Study the drawing (mm; zero at the part's minimum x, y, z) and answer. A direction names the side the tool comes from. Round coordinates to 2 decimals unless told otherwise and drop trailing zeros. Write each loop counter-clockwise with the first axis right and the second up, starting at its lowest first coordinate (ties: lowest second). Pieces come first, ordered by that corner, then holes. Notation, with made-up numbers: (-34.5, 71.25) - (-2.5, 71.25) arc R20 ccw to (-2.5, 107.25) - close; hole circle Ø1 at (75, 6). An arc over 180 degrees is marked (long way). Use one line per item in the form item = value. Start each with the question number.
1) The part is cut by section C-C, the plane x = 1.1. Give the vertices of the cut face in (y, z).
2) The part is cut by section D-D, the plane y = 0.7. Give the vertices of the cut face in (x, z), plus the area to 3 significant figures.
3) For the marked faces 5, 6 and 7, determine the directions among +Z, -Z, +X, -X, +Y, -Y from which every point of the face is accessible in a straight line to the end or side of a thin tool.
4) The part is cut by section B-B, the plane y = 1.25. Give the vertices of the cut face in (x, z) (3 decimals), plus the area to 3 significant figures.
5) The part is cut by section A-A, the plane z = 1. Give the vertices of the cut face in (x, y) (3 decimals), plus the area to 3 significant figures.
6) Consider line 1 along Z through (x, y) = (2.7, 1.2); line 2 along Z through (x, y) = (3.45, 1.9); line 3 along X through (y, z) = (1.15, 2.5). Determine where each line is inside the solid, lowest interval first. Write a range as from..to.
7) For a pull along X with two mould halves and no side action, classify the marked faces 1, 2, 3 and 4 as released by +X, released by -X, zero draft, split by the parting line, or undercut.
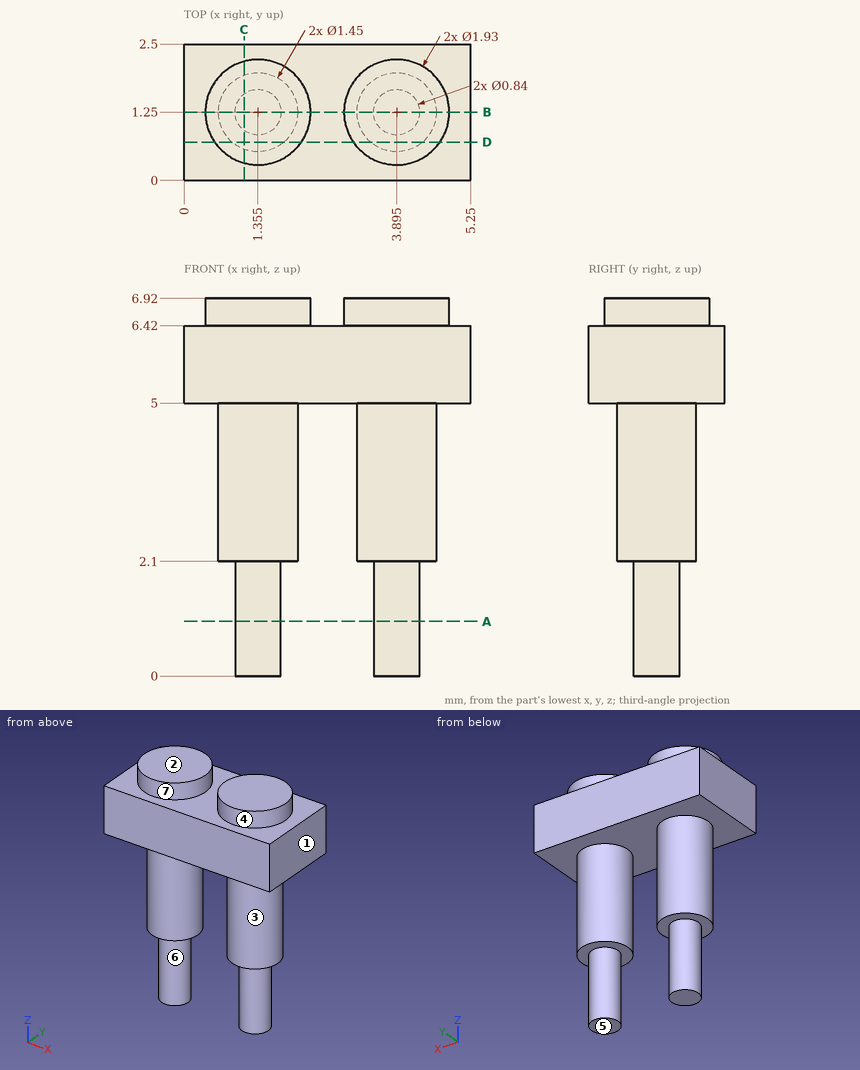
Geometry results:
q1.outline = (0, 5) - (0.57, 5) - (0.57, 2.1) - (0.92, 2.1) - (0.92, 0) - (1.58, 0) - (1.58, 2.1) - (1.93, 2.1) - (1.93, 5) - (2.5, 5) - (2.5, 6.42) - (2.18, 6.42) - (2.18, 6.92) - (0.32, 6.92) - (0.32, 6.42) - (0, 6.42) - close
q2.outline = (0, 5) - (0.88, 5) - (0.88, 2.1) - (1.83, 2.1) - (1.83, 5) - (3.42, 5) - (3.42, 2.1) - (4.37, 2.1) - (4.37, 5) - (5.25, 5) - (5.25, 6.42) - (4.69, 6.42) - (4.69, 6.92) - (3.1, 6.92) - (3.1, 6.42) - (2.15, 6.42) - (2.15, 6.92) - (0.56, 6.92) - (0.56, 6.42) - (0, 6.42) - close
q2.area = 14.5 mm2
q3.face_5 = -Z, +X, -X, +Y, -Y
q3.face_6 = -Z
q3.face_7 = +Z
q4.outline = (0, 5) - (0.63, 5) - (0.63, 2.1) - (0.935, 2.1) - (0.935, 0) - (1.775, 0) - (1.775, 2.1) - (2.08, 2.1) - (2.08, 5) - (3.17, 5) - (3.17, 2.1) - (3.475, 2.1) - (3.475, 0) - (4.315, 0) - (4.315, 2.1) - (4.62, 2.1) - (4.62, 5) - (5.25, 5) - (5.25, 6.42) - (4.86, 6.42) - (4.86, 6.92) - (2.93, 6.92) - (2.93, 6.42) - (2.32, 6.42) - (2.32, 6.92) - (0.39, 6.92) - (0.39, 6.42) - (0, 6.42) - close
q4.area = 21.3 mm2
q5.outline = circle Ø0.84 at (1.355, 1.25); circle Ø0.84 at (3.895, 1.25)
q5.area = 1.11 mm2
q6.line_1 = 5..6.42
q6.line_2 = 5..6.92
q6.line_3 = 0.64..2.07, 3.18..4.61
q7.face_1 = released by +X
q7.face_2 = zero draft
q7.face_3 = undercut
q7.face_4 = undercut
